from build123d import *

# Parameters (mm, degrees)
F1_DEPTH = 1.27
F0_R     = 1.1698918357
F0_R_2   = 1.149683984
F2_DEPTH = 2.286


with BuildPart() as f1:
    # F0 (on Front) → F1 (new body)
    with BuildSketch(Plane.XZ):
        Polygon((-15.388094912, 1.7704545665), (-15.388094912, 16.057066756), (-15.388094912, 16.8387157017), (-30.0930766836, 19.0700641461), (-30.0930766836, 18.4871374451), (-30.0930766836, 4.9859051822), align=None)
        Polygon((-28.1987807881, 11.4603284719), (-17.8684613835, 9.9950339617), (-17.5021312367, 3.694271666), (-28.1987807881, 5.9654787155), align=None, mode=Mode.SUBTRACT)
        Polygon((-27.7591816317, 12.9256220507), (-27.7591816317, 17.9808847578), (-17.5021312367, 16.3690615418), (-17.5021312367, 11.6068571778), align=None, mode=Mode.SUBTRACT)
    extrude(amount=F1_DEPTH)



with BuildPart() as f1b:
    # F0 (on Front) → F1, piece 2 (new body)
    with BuildSketch(Plane.XZ):
        Polygon((-18.2767084967, 15.855339353), (-27.1837434899, 17.1943055438), (-27.1837434899, 13.5655133026), (-18.2767084967, 12.5176263945), align=None)
        with Locations((-22.6742944847, 14.9233993115)):
            Circle(F0_R, mode=Mode.SUBTRACT)
    extrude(amount=F1_DEPTH)


with BuildPart() as f1c:
    # F0 (on Front) → F1, piece 3 (new body)
    with BuildSketch(Plane.XZ):
        Polygon((-30.6900013238, 19.9313648045), (-15.4686479767, 17.6216616277), (-1.8903917537, 21.5964431966), (-17.1117451009, 23.9061463734), align=None)
    extrude(amount=F1_DEPTH)


with BuildPart() as f1d:
    # F0 (on Front) → F1, piece 4 (new body)
    with BuildSketch(Plane.XZ):
        Polygon((-14.626094912, 16.057066756), (-14.626094912, 1.9935158717), (-3.9594611633, 5.1159742), (-3.9594611633, 19.5436675764), (-3.9680227461, 20.1817290912), (-14.626094912, 17.0617770069), align=None)
    extrude(amount=F1_DEPTH)


with BuildPart() as f1e:
    # F0 (on Front) → F1, piece 5 (new body)
    with BuildSketch(Plane.XZ):
        Polygon((-3.8323173759, 4.3592156278), (-14.626094912, 1.1995383243), (-14.626094912, -2.6566980141), (-13.0292281976, -2.3633678097), (-13.0292281976, -1.1240722508), (-13.0411074846, -0.5566334484), (-12.4813056802, -0.3927618984), (-6.0969826496, 1.4761297395), (-5.1597074379, 1.7504995978), (-4.9214556754, 1.0262658156), (-4.9214556754, 0.4425999067), (-3.7855914693, 0.7751029937), align=None)
    extrude(amount=F1_DEPTH)


with BuildPart() as f1f:
    # F0 (on Front) → F1, piece 6 (new body)
    with BuildSketch(Plane.XZ):
        Polygon((-15.388094912, -2.7357117464), (-15.388094912, 1.0209244658), (-15.527460836, 1.0209244658), (-30.0231560015, 4.1906116282), (-30.0930766836, 4.2085912157), (-30.0930766836, 0.4284923682), (-27.5556394443, -0.2239908959), (-27.5556394443, 1.4215863233), (-27.0130208861, 1.3366546978), (-20.7008908468, 0.3486688349), (-19.8447576891, 0.273127106), (-19.9932244299, -1.7287355547), align=None)
    extrude(amount=F1_DEPTH)


with BuildPart() as f1g:
    # F0 (on Front) → F1, piece 7 (new body)
    with BuildSketch(Plane.XZ):
        Polygon((-18.5878000389, 9.4085130813), (-27.4529627692, 10.7276812168), (-27.4529627692, 6.66401535), (-18.3046332728, 4.8343520584), align=None)
        with Locations((-22.5763938557, 7.5477305772)):
            Circle(F0_R_2, mode=Mode.SUBTRACT)
    extrude(amount=F1_DEPTH)


with BuildPart() as f1_1:
    add(f1.part)

    add(f1b.part)  # F2 merges F1b

    add(f1c.part)  # F2 merges F1c

    add(f1d.part)  # F2 merges F1d

    add(f1e.part)  # F2 merges F1e

    add(f1f.part)  # F2 merges F1f

    add(f1g.part)  # F2 merges F1g
    # F0 (on Front) → F2 (join)
    with BuildSketch(Plane.XZ):
        Polygon((-17.5021312367, 3.694271666), (-17.8684613835, 9.9950339617), (-28.1987807881, 11.4603284719), (-28.1987807881, 5.9654787155), align=None)
        Polygon((-27.4529627692, 6.66401535), (-27.4529627692, 10.7276812168), (-18.5878000389, 9.4085130813), (-18.3046332728, 4.8343520584), align=None, mode=Mode.SUBTRACT)
        Polygon((-17.5021312367, 16.3690615418), (-27.7591816317, 17.9808847578), (-27.7591816317, 12.9256220507), (-17.5021312367, 11.6068571778), align=None)
        Polygon((-27.1837434899, 13.5655133026), (-27.1837434899, 17.1943055438), (-18.2767084967, 15.855339353), (-18.2767084967, 12.5176263945), align=None, mode=Mode.SUBTRACT)
        Polygon((-32.4763386121, 20.2024253873), (-30.6900013238, 19.9313648045), (-17.1117451009, 23.9061463734), (-1.8903917537, 21.5964431966), (-0.1563745312, 22.1040444366), (-1.7350990934, 22.3436016595), (-17.1640651666, 24.6848081963), (-28.1764094956, 21.4611495356), align=None)
        Polygon((-3.9594611633, 5.1159742), (-14.626094912, 1.9935158717), (-14.626094912, 1.7704545955), (-14.626094912, 1.1995383243), (-3.8323173759, 4.3592156278), (-3.7855914693, 0.7751029937), (-3.0450882633, 0.9918715129), (-3.1974611633, 4.7442035481), (-3.1974611633, 19.5436675764), (-3.1974611633, 20.4072966403), (-3.9680227461, 20.1817290912), (-3.9594611633, 19.5436675764), align=None)
        Polygon((-30.0930766836, 4.2085912157), (-30.0930766836, 4.9859051822), (-30.0930766836, 18.4871374451), (-30.0930766836, 19.0700641461), (-30.8550766836, 19.185690778), (-30.8550766836, 18.4871374451), (-30.8550766836, 4.9331725397), (-30.8550766836, 0.6244350459), (-30.8505439091, 0.6232694764), (-30.8485884176, 0.6227666362), (-30.0930766836, 0.4284923682), align=None)
        Polygon((-30.0930766836, 19.0700641461), (-15.388094912, 16.8387157017), (-15.4686479767, 17.6216616277), (-30.6900013238, 19.9313648045), (-32.4763386121, 20.2024253873), (-32.3898017041, 19.4185714671), (-30.8550766836, 19.185690778), align=None)
        Polygon((-15.4686479767, 17.6216616277), (-15.388094912, 16.8387157017), (-14.626094912, 17.0617770069), (-3.9680227461, 20.1817290912), (-3.1974611633, 20.4072966403), (-0.1563745312, 21.2975181015), (-0.1563745312, 22.1040444366), (-1.8903917537, 21.5964431966), align=None)
        Polygon((-15.388094912, 16.8387157017), (-15.388094912, 16.057066756), (-15.388094912, 1.7704545665), (-14.626094912, 1.9935158717), (-14.626094912, 16.057066756), (-14.626094912, 17.0617770069), align=None)
        Polygon((-15.388094912, 1.0209244658), (-15.388094912, 1.7704545665), (-30.0930766836, 4.9859051822), (-30.0930766836, 4.2085912157), (-30.0231560015, 4.1906116282), (-15.527460836, 1.0209244658), align=None)
        Polygon((-13.0292281976, -1.1240722508), (-13.0292281976, -2.3633678097), (-12.4034496222, -2.2484178544), (-12.2672281976, -2.223395191), (-12.2672281976, -1.1240722507), (-5.880947848, 0.7453923558), (-4.9214556754, 1.0262658156), (-5.1597074379, 1.7504995978), (-6.0969826496, 1.4761297395), (-12.4813056802, -0.3927618984), (-13.0411074846, -0.5566334484), align=None)
        Polygon((-20.7515549942, -0.414678788), (-20.7008908468, 0.3486688349), (-27.0130208861, 1.3366546978), (-27.0130208861, 0.5653770321), align=None)
        with Locations((-22.6742944847, 14.9233993115)):
            Circle(F0_R)
        with Locations((-22.5763938557, 7.5477305772)):
            Circle(F0_R_2)
        Polygon((-15.388094912, -2.7966706329), (-15.388094912, -2.7357117464), (-19.9932244299, -1.7287355547), (-20.0464328287, -2.4461750717), (-15.388094912, -3.57141984), (-15.388094912, -2.8208797925), (-15.5198876856, -2.8208797925), align=None)
        Polygon((-15.1740174294, 1.0391442142), (-15.388094912, 1.0209244658), (-15.388094912, -2.7357117464), (-15.388094912, -2.7966706329), (-14.626094912, -2.6566980141), (-14.626094912, 1.1995383243), align=None)
        Polygon((-27.5556394443, -0.2239908959), (-30.0930766836, 0.4284923682), (-30.0930766836, -0.1490246532), (-30.0930766836, -0.3582970146), (-27.5556394443, -1.0107802787), align=None)
        Polygon((-20.8266744405, -1.5464900143), (-19.9932244299, -1.7287355547), (-19.8447576891, 0.273127106), (-20.7008908468, 0.3486688349), (-20.7515549942, -0.414678788), (-20.7364695061, -0.4170399955), (-20.7708697434, -0.7056906514), align=None)
        Polygon((-13.0292281976, -2.3633678097), (-14.626094912, -2.6566980141), (-14.626094912, -3.4314472213), (-13.0292281976, -3.1381170169), (-13.0292281976, -2.9902135849), align=None)
        Polygon((-3.0450882633, 0.9918715129), (-3.7855914693, 0.7751029937), (-4.9214556754, 0.4425999067), (-4.9214556754, -0.2108097675), (-3.0450882633, 0.3384618388), align=None)
        Polygon((-4.9214556754, -0.2108097675), (-4.9214556754, 0.4425999067), (-4.9214556754, 1.0262658156), (-5.880947848, 0.7453923558), (-5.8803612014, -0.4915114974), align=None)
        Polygon((-27.5556394443, 1.4215863233), (-27.5556394443, -0.2239908959), (-27.0130208861, -0.3635212545), (-27.0130208861, 0.5396492752), (-27.0484225739, 0.5709181675), (-27.0130208861, 0.5653770321), (-27.0130208861, 1.3366546978), align=None)
        Polygon((-14.626094912, 1.9935158717), (-15.388094912, 1.7704545665), (-15.388094912, 1.0209244658), (-15.1740174294, 1.0391442142), (-14.626094912, 1.1995383243), (-14.626094912, 1.7704545955), align=None)
        Polygon((-30.0930766836, -0.1490246532), (-30.0930766836, 0.4284923682), (-30.8485884176, 0.6227666362), (-30.8505439091, 0.6232694764), (-30.8550766836, 0.6244350459), (-30.8550766836, -0.1623543369), (-30.0930766836, -0.3582970146), align=None)
        Polygon((-20.0464328287, -2.4461750717), (-19.9932244299, -1.7287355547), (-20.8266744405, -1.5464900143), (-20.8731335697, -2.2464813826), align=None)
        Polygon((-14.626094912, -2.6566980141), (-15.388094912, -2.7966706329), (-15.388094912, -2.8208797925), (-15.388094912, -3.57141984), (-14.6509673791, -3.4360160722), (-14.626094912, -3.4314472213), align=None)
        Polygon((-12.4034496222, -2.2484178544), (-13.0292281976, -2.3633678097), (-13.0292281976, -2.9902135849), (-13.0292281976, -3.1381170169), (-12.2672281976, -2.9981443981), (-12.2672281976, -2.223395191), align=None)
        Polygon((-27.0130208861, -0.3635212545), (-27.5556394443, -0.2239908959), (-27.5556394443, -1.0107802787), (-27.0130208861, -1.1503106373), (-27.0130208861, -0.3672745107), align=None)
    extrude(amount=F2_DEPTH)


solid = f1_1.part
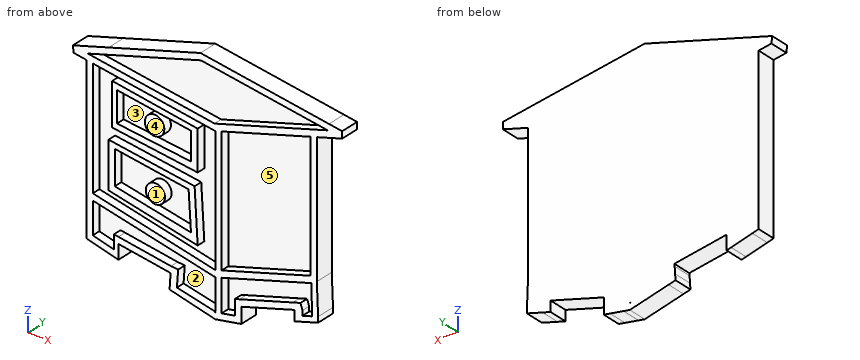
The model under review builds one solid part; all positions refer to its coordinate system, in mm. Face numbers are marked on the shaded views. A direction names the side the tool comes from. Coordinates: 2 decimals unless noted, no trailing zeros. Loops run counter-clockwise (first coordinate to the right, second up) from the corner with the lowest first, then second, coordinate; pieces in that order, holes last. Notation, with made-up numbers: M 55.25,7.25 L 76.25,7.25 A10 ccw 76.25,24.25 Z; hole C 72.25,51 d3. An arc over 180 degrees is marked long. Put each result on its own line as item: value. Start each with the question number.
Q1. Add section A-A (x = -10). Write out the cut boundary in (y, z), and give its area (3 significant figures).
Q2. The part is to be moulded in two halves that separate along Z. For the marked faces 1, 2 and 3, say which applies: +Z half, -Z half, draft (parallel to the pull), parting line (faces both ways), or undercut.
Q3. Clearance check with flat-ended pins moving along their axes: pin 1 (1.1 mm diameter, centred on y = -1.5, z = 0, fed in from -X); pin 2 (3 mm diameter, centred on x = -24.5, z = 8, fed in from -Y); pin 3 (0.5 mm diameter, centred on y = -1.5, z = 1, fed in from +X); pin 4 (0.8 mm diameter, centred on y = -1.5, z = 2, fed in from +X). State where each tip first meets the part, or that it passes through.
Q4. For the marked faces 4 and 5, list the 3-axis set-ups (+Z, -Z, +X, -X, +Y, -Y) from which the entire face can be reached by the end or side of a thin tool; tool diameter is ignored.
Q5. Wall thickness on line 1 (Z direction, x = -4.5, y = -1.8); line 2 (Z direction, x = -8, y = -1.75); line 3 (Y direction, x = -4.5, z = 16.75): over which ranges is each line inside the solid? List them lowest first.
Q6. Add section B-B (z = 23.25). Write out the cut boundary in (x, y), and give its area (3 significant figures).
Answers:
1. outline: M -2.29,-0.46 L 0,-0.46 L 0,23.6 L -2.29,23.6 L -2.29,22.83 L -1.27,22.83 L -1.27,19.22 L -2.29,19.22 L -2.29,18.42 L -1.27,18.42 L -1.27,3.35 L -2.29,3.35 L -2.29,2.55 L -1.27,2.55 L -1.27,0.33 L -2.29,0.33 Z
1. area: 33.8 mm^2
2. face 1: draft
2. face 2: undercut
2. face 3: undercut
3. pin 1: stops at x = -30.86
3. pin 2: stops at y = -2.29
3. pin 3: stops at x = -3.05
3. pin 4: stops at x = -3.07
4. face 4: +Z, -Z, +X, -X, -Y
4. face 5: -Y
5. line 1: z = -0.09 to 0.57, 4.16 to 4.96, 20.03 to 20.83, 21.99 to 22.76
5. line 2: z = 0.13 to 0.92, 3.14 to 3.93, 19 to 19.81, 22.52 to 23.29
5. line 3: y = -1.27 to 0
6. outline: M -22.07,-2.29 L -19.35,-2.29 L -19.35,-1.27 L -12.79,-1.27 L -12.79,-2.29 L -7.71,-2.29 L -7.71,0 L -22.07,0 Z
6. area: 26.1 mm^2
